Verification items for the finished model (mm, model axes). A direction names the side the tool comes from. Give positions to 0.01 mm unless a question says otherwise; leave off trailing zeros. Order: outer loops, then holes, each group sorted by start corner. A loop starts at its lowest first (then second) coordinate and runs counter-clockwise, first axis right, second up. Notation, with made-up numbers: (56.5, 12) -> (64.5, 12) arc R9 cw to (64.5, 24) -> close; hole circle Ø2 at (68, 46.5). An arc over 180 degrees is marked (long way). Write each question's results on one line, items separated by ' | '. Start each with the question number.
1. Cross-section at A-A, the plane y = -3.5. Enter the section's corners in (x, z).
2. Cross-section at B-B, the plane x = -1.5. Enter the section's corners in (y, z).
3. Cross-section at D-D, the plane y = -7.25. Enter the section's corners in (x, z), then the cut area to 3 significant figures.
4. Cross-section at C-C, the plane z = -0.75. Enter the section's corners in (x, y).
5. Material ranges on L1, parallel to Y at x = 4.5, z = -0.5; L2, parallel to Z at x = 1.5, y = -14; L3, parallel to Z at x = -1.75, y = -2, recorded low to high. Write a range as from..to.
6. Set-up check for faces 1 (the face through (3.209, -1.972, -4.467)), 2 (the face through (-3.746, -10.902, 0.165)): record each of +Z, -Z, +X, -X, +Y, -Y from which the full face is reachable in a straight line by a thin tool's end or side.
7. Depth check by flat-ended pin: pin 1 Ø2 at (y, z) = (-8.5, -0.5) entering from -X; pin 2 Ø5 at (x, y) = (-4.5, -8) entering from -Z; pin 3 Ø5 at (y, z) = (-10.5, -2.5) entering from +X. Enter the tip coordinate at first touch or a pass-through.
from build123d import *

# Parameters (mm, degrees)
F1_DEPTH = 4
F2_R     = 3.75
F3_DEPTH = 14


# Not quite as in the source:
# - a feature names something its author has since deleted; it is built from what else it names


with BuildPart() as f1:
    # F0 (on Front) → F1 (new body)
    with BuildSketch(Plane.XZ):
        Polygon((0.6816548843, -6.3141650241), (5.8090547568, -2.5667520656), (5.1273998724, 3.7474129585), (-0.6816548843, 6.3141650241), (-5.8090547568, 2.5667520656), (-5.1273998724, -3.7474129585), align=None)
    extrude(amount=F1_DEPTH)

    # F2 (on face) → F3 (join)
    with BuildSketch(Plane.XZ.offset(4)):
        Circle(F2_R)
    extrude(amount=F3_DEPTH)


solid = f1.part
Results below:
1) outline: (-5.81, 2.57) -> (-5.13, -3.75) -> (0.68, -6.31) -> (5.81, -2.57) -> (5.13, 3.75) -> (-0.68, 6.31) -> close
2) outline: (-18, -3.44) -> (-4, -3.44) -> (-4, -5.35) -> (0, -5.35) -> (0, 5.72) -> (-4, 5.72) -> (-4, 3.44) -> (-18, 3.44) -> close
3) outline: circle Ø7.5 at (0, 0) | area: 44.2 mm²
4) outline: (-5.45, -4) -> (-3.67, -4) -> (-3.67, -18) -> (3.67, -18) -> (3.67, -4) -> (5.61, -4) -> (5.61, 0) -> (-5.45, 0) -> close
5) L1: y = -4..0 | L2: z = -3.44..3.44 | L3: z = -5.24..5.53
6) face 1: -Z, +X, +Y, -Y | face 2: -Y
7) pin 1: stops at x = -3.75 | pin 2: stops at z = -3.17 | pin 3: stops at x = 3.75
